The figure shows three views and two pictorial views of one solid part (mm, origin at its lowest corner). Answer the questions. Coordinates: 2 decimals unless noted, no trailing zeros. Write each loop counter-clockwise with the first axis right and the second up, starting at its lowest first coordinate (ties: lowest second). Pieces come first, ordered by that corner, then holes. Notation, with made-up numbers: M 71,57 L 122,57 A17 cw 122,85 Z; hole C 5.25,-34 d4. An arc over 180 degrees is marked long. Answer as CSV lines item,"result".
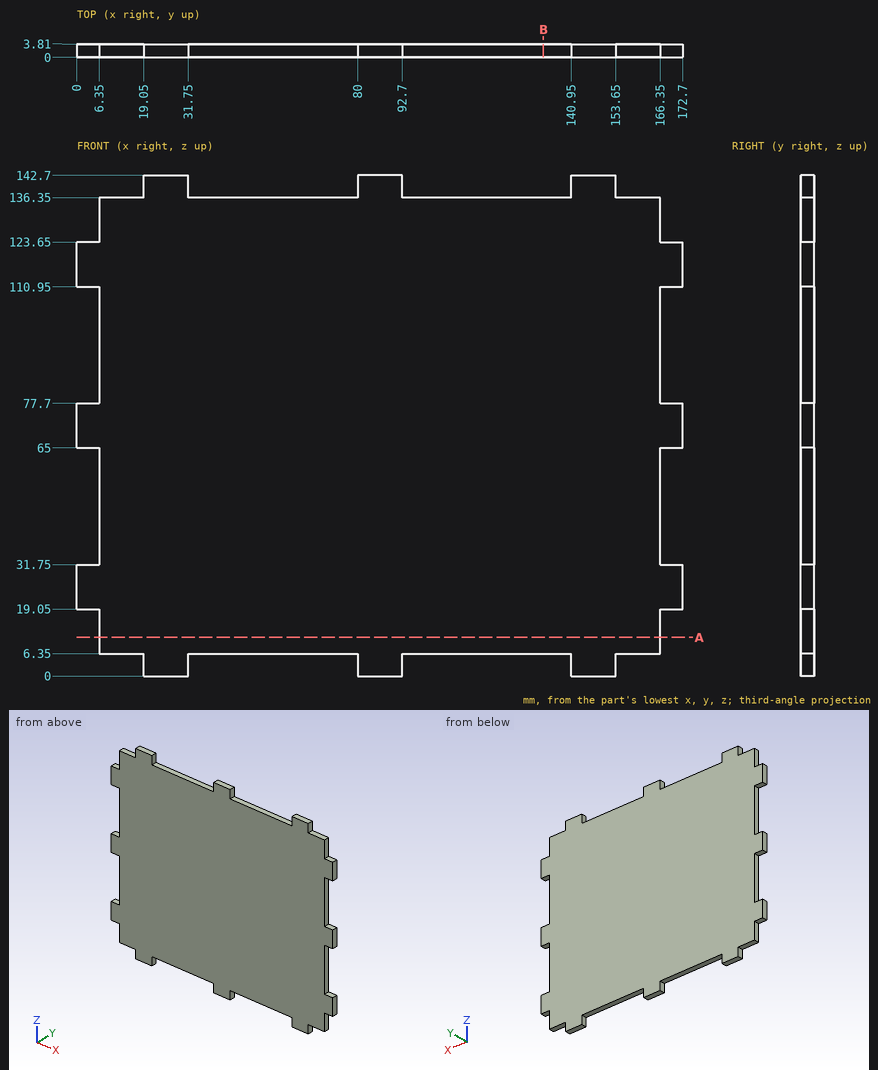
Q1. Find section B-B (x = 133). Give the vertices of the cut face in (y, z).
Output:
outline,"M 0,6.35 L 3.81,6.35 L 3.81,136.35 L 0,136.35 Z"
Q2. Straight lines are drawn through the part: line 1 (Z direction, x = 39.5, y = 1.85); line 2 (X direction, y = 3.6, z = 132). For each, find the intervals that lie inside material, in ascending order.
Output:
line 1,"6.35 to 136.35"
line 2,"6.35 to 166.35"
Q3. Flat-ended cylindrical pins translate along their axes: pin 1 Ø2 at (y, z) = (2.5, 127.5) entering from -X; pin 2 Ø1.1 at (y, z) = (2, 87) entering from -X; pin 3 Ø1.1 at (x, y) = (171, 1.5) entering from +Z; pin 4 Ø3 at (x, z) = (60.5, 118.5) entering from -Y. Find the tip coordinate at first contact, or state that the pin passes through.
Output:
pin 1,"x = 6.35"
pin 2,"x = 6.35"
pin 3,"z = 123.65"
pin 4,"y = 0"
Q4. Find section A-A (z = 11). Give the vertices of the cut face in (x, y), and give its area (3 significant figures).
Output:
outline,"M 6.35,0 L 166.35,0 L 166.35,3.81 L 6.35,3.81 Z"
area,"610 mm2"
